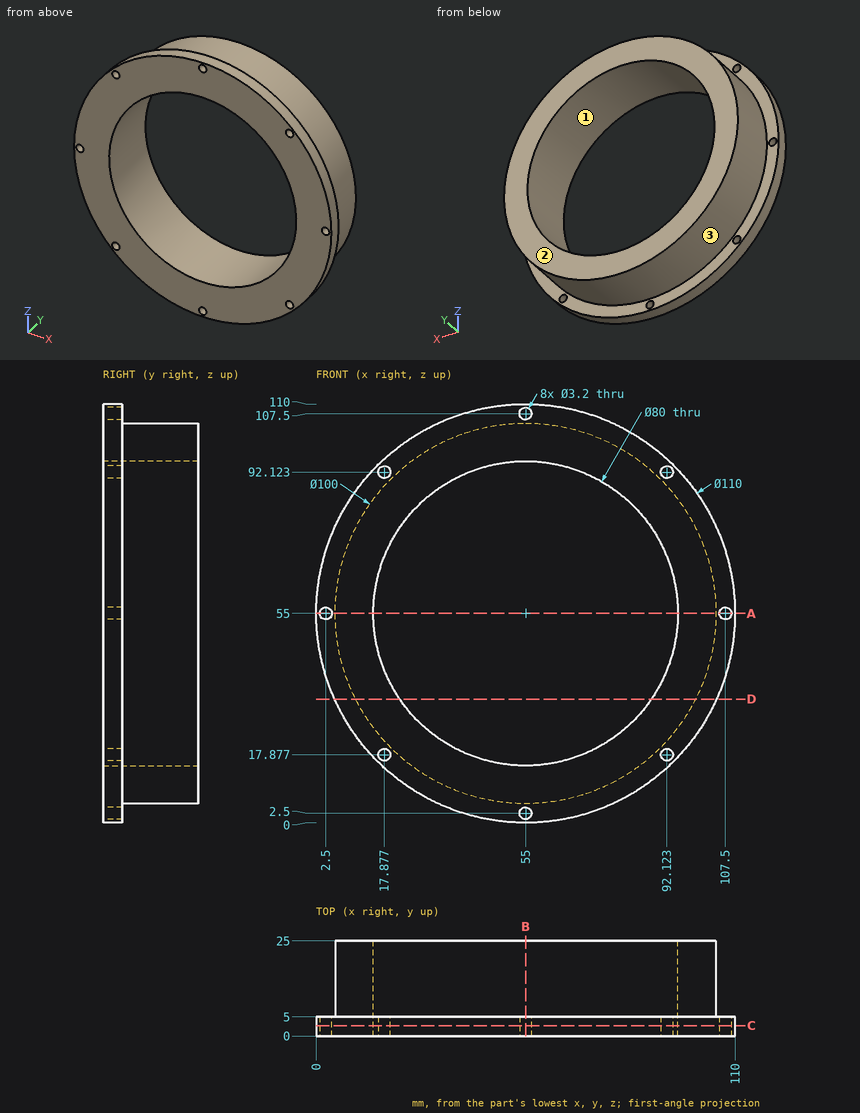
Design review of the part shown in the three views and the two pictorial views. Dimensions are in mm from the part's minimum x, y and z. Round coordinates to 2 decimals unless told otherwise and drop trailing zeros. Write each loop counter-clockwise with the first axis right and the second up, starting at its lowest first coordinate (ties: lowest second). Pieces come first, ordered by that corner, then holes. Notation, with made-up numbers: (43, 75.25) -> (102, 75.25) arc R12 cw to (102, 98.25) -> close; hole circle Ø7 at (33, 61). An arc over 180 degrees is marked (long way). Answer as a JSON object with one key per item and string values.
1. Clearance check with flat-ended pins moving along their axes: pin 1 (1.5 mm diameter, centred on x = 19, y = 11, fed in from +Z); pin 2 (3.5 mm diameter, centred on x = 55, z = 107.5, fed in from +Y); pin 3 (10 mm diameter, centred on x = 51.5, y = 18, fed in from +Z). State where each tip first meets the part, or that it passes through.
Results found:
{"pin 1": "stops at z = 90.46", "pin 2": "stops at y = 5", "pin 3": "stops at z = 105"}
2. We need section B-B on x = 55. State the section outline as (y, z) points.
Results found:
{"outline": "(0, 0) -> (5, 0) -> (5, 0.9) -> (0, 0.9) -> close; (0, 4.1) -> (5, 4.1) -> (5, 5) -> (25, 5) -> (25, 15) -> (0, 15) -> close; (0, 95) -> (25, 95) -> (25, 105) -> (5, 105) -> (5, 105.9) -> (0, 105.9) -> close; (0, 109.1) -> (5, 109.1) -> (5, 110) -> (0, 110) -> close"}
3. To check wall thickness, follow line 1 along X through (y, z) = (7.5, 55); line 2 along X through (y, z) = (4, 53); line 3 along Z through (x, y) = (66, 22.25) (1 decimal). State the ranges of each line that lie inside material, in increasing order.
Results found:
{"line 1": "x = 5 to 15, 95 to 105", "line 2": "x = 0.04 to 15.05, 94.95 to 109.96", "line 3": "z = 6.2 to 16.5, 93.5 to 103.8"}
4. We need section D-D on z = 32.5. State the section outline as (x, y) points, and give its area (3 significant figures).
Results found:
{"outline": "(4.81, 0) -> (21.93, 0) -> (21.93, 25) -> (10.35, 25) -> (10.35, 5) -> (4.81, 5) -> close; (88.07, 0) -> (105.19, 0) -> (105.19, 5) -> (99.65, 5) -> (99.65, 25) -> (88.07, 25) -> close", "area": "634 mm^2"}
5. We need section C-C on y = 2.75. State how many separate pieces and enclosed holes the cut face has, and give its area (3 significant figures).
Results found:
{"separate pieces": "1", "enclosed holes": "9", "area": "4,410 mm^2"}
6. We need section A-A on z = 55. State the section outline as (x, y) points.
Results found:
{"outline": "(0, 0) -> (0.9, 0) -> (0.9, 5) -> (0, 5) -> close; (4.1, 0) -> (15, 0) -> (15, 25) -> (5, 25) -> (5, 5) -> (4.1, 5) -> close; (95, 0) -> (105.9, 0) -> (105.9, 5) -> (105, 5) -> (105, 25) -> (95, 25) -> close; (109.1, 0) -> (110, 0) -> (110, 5) -> (109.1, 5) -> close"}
7. The part is to be moulded in two halves that separate along X. For the marked faces 1, 2 and 3, say which applies: pulls with the +X half, pulls with the -X half, needs draft (parallel to the pull), parting line crosses it, or undercut.
Results found:
{"face 1": "undercut", "face 2": "needs draft", "face 3": "parting line crosses it"}
